from build123d import *

# Parameters (mm, degrees)
F0_W     = 25
F0_H     = 65
F0_W_2   = 13
F0_H_2   = 23
F1_DEPTH = 4
F4_D     = 1
F5_R     = 1


with BuildPart() as f1:
    # F0 (on Top) → F1 (new body)
    with BuildSketch(Plane.XY):
        Rectangle(F0_W, F0_H)
        with Locations((0, -17)):
            Rectangle(F0_W_2, F0_H_2, mode=Mode.SUBTRACT)
        with Locations((0, 17)):
            Rectangle(F0_W_2, F0_H_2, mode=Mode.SUBTRACT)
    extrude(amount=F1_DEPTH)

    # F4 (through all)
    with Locations(Plane(origin=(0, 0, 0), x_dir=(1, 0, 0), z_dir=(0, 0, -1))):
        with Locations((0, 30.5), (0, 3), (0, -3), (0, -30.5)):
            Hole(F4_D / 2)

    # F5
    f5_edges = [f1.edges().sort_by_distance(p)[0] for p in [
        (-12.5, 32.5, 2),
        (12.5, 32.5, 2),
        (-12.5, -32.5, 2),
        (12.5, -32.5, 2),
    ]]
    fillet(f5_edges, radius=F5_R)


solid = f1.part
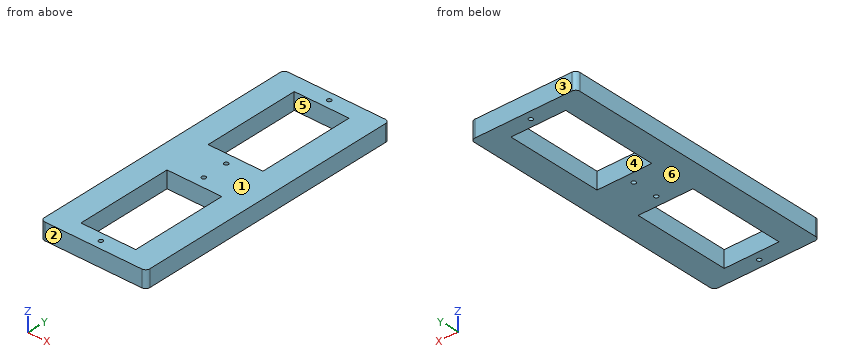
Model file for the job. Use its own axes, mm. Face numbers are marked on the shaded views. A direction names the side the tool comes from. Round coordinates to 2 decimals unless told otherwise and drop trailing zeros. Loops run counter-clockwise (first coordinate to the right, second up) from the corner with the lowest first, then second, coordinate; pieces in that order, holes last. Notation, with made-up numbers: M -32,-7 L -11,-7 A19 ccw -11,18 Z; hole C 43,-5.75 d11. An arc over 180 degrees is marked long. One line per question, with ' | ' between items.
1) Mould opens along Y. For the marked faces 1, 2, 3 and 4 say: +Y half, -Y half, draft (parallel to the pull), parting line (faces both ways), or undercut.
Solved:
face 1: draft | face 2: -Y half | face 3: +Y half | face 4: undercut
2) Band-saw the part on B-B (z = 1.4). Give the cut face in (x, y), then the cut area to 3 significant figures.
Solved:
outline: M -12.5,-31.5 A1 ccw -11.5,-32.5 L 11.5,-32.5 A1 ccw 12.5,-31.5 L 12.5,31.5 A1 ccw 11.5,32.5 L -11.5,32.5 A1 ccw -12.5,31.5 Z; hole M -6.5,-28.5 L 6.5,-28.5 L 6.5,-5.5 L -6.5,-5.5 Z; hole M -6.5,5.5 L 6.5,5.5 L 6.5,28.5 L -6.5,28.5 Z; hole C 0,-30.5 d1; hole C 0,-3 d1; hole C 0,3 d1; hole C 0,30.5 d1 | area: 1,020 mm²
3) Band-saw the part on A-A (y = 19). Give the cut face in (x, z), then the cut area to 3 significant figures.
Solved:
outline: M -12.5,0 L -6.5,0 L -6.5,4 L -12.5,4 Z; M 6.5,0 L 12.5,0 L 12.5,4 L 6.5,4 Z | area: 48.0 mm²
4) 3-axis set-ups, long thin cutter, end or side, ignore diameter. For the marked faces 5 and 6: which of +Z, -Z, +X, -X, +Y, -Y reach the whole face in a straight line?
Solved:
face 5: +Z, -Z | face 6: -Z, +X, -X, +Y, -Y
5) Band-saw the part on C-C (x = 2.5). Give the cut face in (y, z), then the cut area to 3 significant figures.
Solved:
outline: M -32.5,0 L -28.5,0 L -28.5,4 L -32.5,4 Z; M -5.5,0 L 5.5,0 L 5.5,4 L -5.5,4 Z; M 28.5,0 L 32.5,0 L 32.5,4 L 28.5,4 Z | area: 76.0 mm²
6) Drill centre lines: line 1 along Y through (x, z) = (3.5, 2.5); line 2 along X through (y, z) = (3, 2.1); line 3 along X through (y, z) = (6, 0.4). Where is each one in solid material? Low to high.
Solved:
line 1: y = -32.5 to -28.5, -5.5 to 5.5, 28.5 to 32.5 | line 2: x = -12.5 to -0.5, 0.5 to 12.5 | line 3: x = -12.5 to -6.5, 6.5 to 12.5
